Build history of the part. All positions in model axes, mm. Face numbers are marked on the shaded views. A direction names the side the tool comes from. Round coordinates to 2 decimals unless told otherwise and drop trailing zeros. Write each loop counter-clockwise with the first axis right and the second up, starting at its lowest first coordinate (ties: lowest second). Pieces come first, ordered by that corner, then holes. Notation, with made-up numbers: (-19, 72) -> (25, 72) arc R17 ccw to (25, 82) -> close; hole circle Ø2 at (37.5, 84.5). An arc over 180 degrees is marked (long way). Answer in a Markdown table with one row per item.
```python
from build123d import *

# Parameters (mm, degrees)
SKETCH2_R          = 5.1435
EXTRUDE1_DEPTH     = 7.112
EXTRUDE1_TAPER     = -1.5
SKETCH5_OUTSIDE_W  = 32.218
SKETCH5_OUTSIDE_H  = 32.218
SKETCH5_OUTSIDE_R  = 4.532470965
CUT_EXTRUDE1_DEPTH = 8.1120001
CUT_EXTRUDE1_TAPER = 45
SKETCH9_OUTSIDE_W  = 15.994
SKETCH9_OUTSIDE_H  = 15.994
SKETCH9_OUTSIDE_R  = 4.532470965
CUT_EXTRUDE5_DEPTH = 0.376296296
SKETCH10_OUTSIDE_W = 31.44
SKETCH10_OUTSIDE_H = 31.44
SKETCH10_OUTSIDE_R = 4.532470965
CUT_EXTRUDE6_DEPTH = 7.735703804
CUT_EXTRUDE6_TAPER = 45
CUT_EXTRUDE7_DEPTH = 2.286
CHAMFER1_SIZE      = 0.254
SKETCH11_R         = 2.749630657
CUT_EXTRUDE8_DEPTH = 2.286
CUT_EXTRUDE8_TAPER = 45


with BuildPart() as part:
    # Sketch2 → Extrude1 (new body)
    with BuildSketch(Plane(origin=(-3.556, 0, 0), x_dir=(0, 0, -1), z_dir=(1, 0, 0))):
        Circle(SKETCH2_R)
    extrude(amount=EXTRUDE1_DEPTH, taper=EXTRUDE1_TAPER)

    # Sketch5 outside → Cut-Extrude1 (cut, through all)
    with BuildSketch(Plane(origin=(-3.556, 0, 0), x_dir=(0, 0, -1), z_dir=(1, 0, 0))):
        Rectangle(SKETCH5_OUTSIDE_W, SKETCH5_OUTSIDE_H)
        Circle(SKETCH5_OUTSIDE_R, mode=Mode.SUBTRACT)
    extrude(amount=CUT_EXTRUDE1_DEPTH, taper=CUT_EXTRUDE1_TAPER, mode=Mode.SUBTRACT)

    # Sketch9 outside → Cut-Extrude5 (cut)
    with BuildSketch(Plane(origin=(3.556, 0, 0), x_dir=(0, 0, -1), z_dir=(1, 0, 0))):
        Rectangle(SKETCH9_OUTSIDE_W, SKETCH9_OUTSIDE_H)
        Circle(SKETCH9_OUTSIDE_R, mode=Mode.SUBTRACT)
    extrude(amount=-CUT_EXTRUDE5_DEPTH, mode=Mode.SUBTRACT)

    # Sketch10 outside → Cut-Extrude6 (cut, through all)
    with BuildSketch(Plane(origin=(3.179703704, 0, 0), x_dir=(0, 0, -1), z_dir=(1, 0, 0))):
        Rectangle(SKETCH10_OUTSIDE_W, SKETCH10_OUTSIDE_H)
        Circle(SKETCH10_OUTSIDE_R, mode=Mode.SUBTRACT)
    extrude(amount=-CUT_EXTRUDE6_DEPTH, taper=CUT_EXTRUDE6_TAPER, mode=Mode.SUBTRACT)

    # Sketch6 → Cut-Extrude7 (cut)
    with BuildSketch(Plane(origin=(3.556, 0, 0), x_dir=(0, 0, -1), z_dir=(1, 0, 0))):
        Polygon((0, 2.749630657), (-2.38125, 1.374815329), (-2.38125, -1.374815329), (0, -2.749630657), (2.38125, -1.374815329), (2.38125, 1.374815329), align=None)
    extrude(amount=-CUT_EXTRUDE7_DEPTH, mode=Mode.SUBTRACT)

    # Chamfer1
    chamfer1_edges = [part.edges().sort_by_distance(p)[0] for p in [
        (3.556, 0, 4.532470965),
    ]]
    chamfer(chamfer1_edges, length=CHAMFER1_SIZE)

    # Sketch11 → Cut-Extrude8 (cut)
    with BuildSketch(Plane(origin=(3.556, 0, 0), x_dir=(0, 0, -1), z_dir=(1, 0, 0))):
        Circle(SKETCH11_R)
    extrude(amount=-CUT_EXTRUDE8_DEPTH, taper=CUT_EXTRUDE8_TAPER, mode=Mode.SUBTRACT)


solid = part.part
```
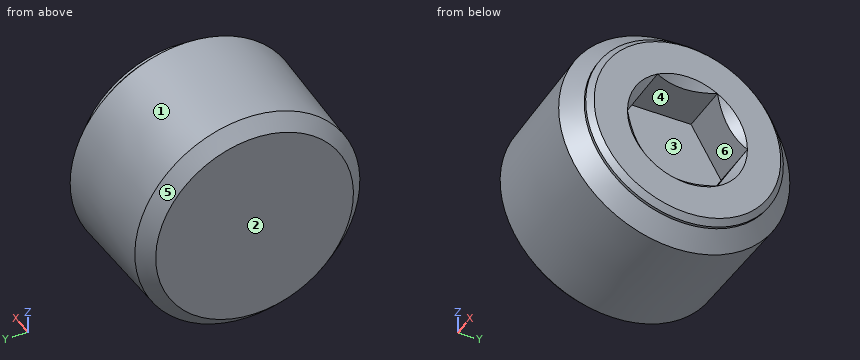
Q1. Saw through at A-A on x = 1.5. Write the cut outline in (y, z), plus the area to 3 significant figures.
A:
| item | result |
|---|---|
| outline | circle Ø10.55 at (0, 0); hole (-2.75, 0) -> (-1.37, -2.38) -> (1.37, -2.38) -> (2.75, 0) -> (1.37, 2.38) -> (-1.37, 2.38) -> close |
| area | 67.8 mm² |
Q2. Drop flat-ended pins along their axis: P1, Ø3, axis at x = -1, z = -0.5, coming from the +Y side; P2, Ø2, axis at x = -2.5, y = -0.5, coming from the +Z side; P3, Ø3, axis at x = -1, y = -3.5, coming from the -Z side. Give the stop position or say it passes through.
A:
| item | result |
|---|---|
| P1 | y = 5.25 |
| P2 | z = 5.19 |
| P3 | z = -4.81 |
Q3. Saw through at B-B on x = -1. Write the cut outline in (y, z).
A:
| item | result |
|---|---|
| outline | circle Ø10.42 at (0, 0) |
Q4. Two-plate mould, pull along Y, no slides. Class the marked faces 1, 2, 3 and 4: released by +Y, released by -Y, zero draft, split by the parting line, or undercut.
A:
| item | result |
|---|---|
| face 1 | split by the parting line |
| face 2 | zero draft |
| face 3 | undercut |
| face 4 | undercut |
Q5. Which spindle directions (+Z, -Z, +X, -X, +Y, -Y) get a long thin tool onto all of the face, cutting with end or side? Do the marked faces 5 and 6. Say none if no direction does.
A:
| item | result |
|---|---|
| face 5 | -X |
| face 6 | +X |
Q6. Wall check: line 1 (X direction, y = -1.25, z = 1.25); line 2 (Z direction, x = 2.5, y = -1.5); line 3 (Z direction, x = 2.75, y = 2.5). Give the ranges that are in metal, low to high. Write a range as [from, to].
A:
| item | result |
|---|---|
| line 1 | [-3.56, 1.27] |
| line 2 | [-4.99, -2.16], [2.16, 4.99] |
| line 3 | [-4.29, -0.43], [0.43, 4.29] |
Q7. Saw through at C-C on x = 3. Write the cut outline in (y, z).
A:
| item | result |
|---|---|
| outline | circle Ø9.42 at (0, 0); hole (-2.75, 0) -> (-1.37, -2.38) -> (1.37, -2.38) -> (2.75, 0) -> (1.37, 2.38) -> (-1.37, 2.38) -> close |
Q8. Saw through at D-D on x = -2. Write the cut outline in (y, z), plus the area to 3 significant figures.
A:
| item | result |
|---|---|
| outline | circle Ø10.37 at (0, 0) |
| area | 84.4 mm² |
